```python
from build123d import *

# Parameters (mm, degrees)
F1_R     = 12.7
F2_DEPTH = 95.25
F0_R     = 63.5
F3_DEPTH = 3.175
F4_R     = 2.54
F6_ANGLE = 30
F7_R     = 63.5
F8_DEPTH = 254


with BuildPart() as f2:
    # F1 (on Top) → F2 (new body, symmetric)
    with BuildSketch(Plane.XY):
        Circle(F1_R)
    extrude(amount=F2_DEPTH, both=True)

    # F0 (on Front) → F3 (join, symmetric)
    with BuildSketch(Plane.XZ):
        Circle(F0_R)
    extrude(amount=F3_DEPTH, both=True)

    # F4
    f4_edges = [f2.edges().sort_by_distance(p)[0] for p in [
        (-63.5, -3.175, 0),
        (63.5, -3.175, 0),
        (-63.5, 3.175, 0),
        (63.5, 3.175, 0),
    ]]
    fillet(f4_edges, radius=F4_R)


with BuildPart() as f2_1:
    # F6: moved
    add(f2.part.rotate(Axis((0, 0, -0.5104467273), (0, 0, -1)), F6_ANGLE))


with BuildPart() as f8:
    # F7 (on Front) → F8 (new body, symmetric)
    with BuildSketch(Plane.XZ):
        Circle(F7_R)
    extrude(amount=F8_DEPTH, both=True)

    # F9: cut F2
    add(f2_1.part, mode=Mode.SUBTRACT)


solid = f8.part
```
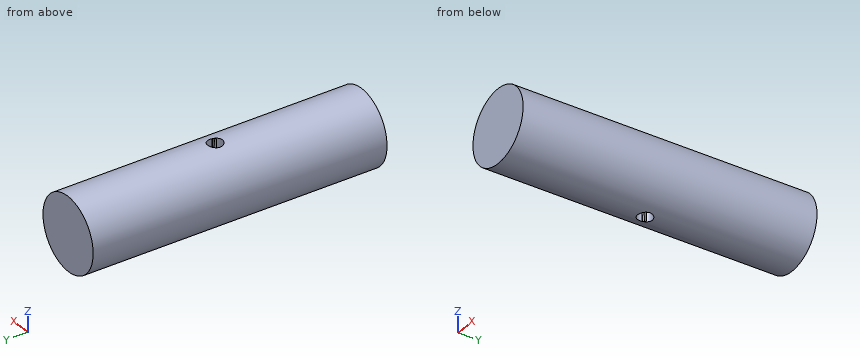
CAD build for the part. Positions are in the model's coordinates, mm. Give positions to 0.01 mm unless a question says otherwise; leave off trailing zeros. Order: outer loops, then holes, each group sorted by start corner. A loop starts at its lowest first (then second) coordinate and runs counter-clockwise, first axis right, second up.
(1) Saw through at C-C, the plane y = -109. Give the cut face in (x, z), then the cut area to 3 significant figures.
(2) Drill centre lines: L1, parallel to Y at x = 0, z = -7; L2, parallel to X at y = -211, z = -1; L3, parallel to Y at x = -53, z = -3.5. Where is each one in solid material? Low to high.
(3) Flat gauge pins, fed straight in: pin 1 (6 mm diameter, centred on y = 155, z = 13.5, fed in from +X); pin 2 (8 mm diameter, centred on x = 40.5, y = -178.5, fed in from +Z); pin 3 (4 mm diameter, centred on y = 84, z = 42.5, fed in from -X). Where does each tip first touch, or does it go through?
(4) Saw through at A-A, the plane z = 0. Give the cut face in (x, y).
(5) Saw through at B-B, the plane x = 0. Give the cut face in (y, z), then the cut area to 3 significant figures.
Results found:
1. outline: circle Ø127 at (0, 0)
1. area: 12,700 mm2
2. L1: y = -254 to -12.7, 12.7 to 254
2. L2: x = -63.49 to 63.49
2. L3: y = -254 to 26.93, 33.45 to 254
3. pin 1: stops at x = 62.63
3. pin 2: stops at z = 51.96
3. pin 3: stops at x = -48.91
4. outline: (-63.5, -254) - (63.5, -254) - (63.5, 254) - (-63.5, 254) - close; hole (-55.31, 31.2) arc R2.54 ccw to (-54.38, 27.73) - (-12.24, 3.4) arc R12.7 ccw to (9.06, -8.9) - (51.21, -33.23) arc R2.54 ccw to (54.68, -32.3) - (55.31, -31.2) arc R2.54 ccw to (54.38, -27.73) - (12.24, -3.4) arc R12.7 ccw to (-9.06, 8.9) - (-51.21, 33.23) arc R2.54 ccw to (-54.68, 32.3) - close
5. outline: (-254, -63.5) - (-12.7, -63.5) - (-12.7, 63.5) - (-254, 63.5) - close; (12.7, -63.5) - (254, -63.5) - (254, 63.5) - (12.7, 63.5) - close
5. area: 61,300 mm2
